Build history of the part. All positions in model axes, mm. Face numbers are marked on the shaded views. A direction names the side the tool comes from. Round coordinates to 2 decimals unless told otherwise and drop trailing zeros. Write each loop counter-clockwise with the first axis right and the second up, starting at its lowest first coordinate (ties: lowest second). Pieces come first, ordered by that corner, then holes. Notation, with made-up numbers: M 10.25,24.5 L 68.25,24.5 A18 ccw 68.25,41.5 Z; hole C -31,-16.75 d5. An arc over 180 degrees is marked long. Write item = value, one per line.
from build123d import *

# Parameters (mm, degrees)
SKETCH1_W           = 80
SKETCH1_H           = 80
BOSS_EXTRUDE1_DEPTH = 60
SKETCH2_W           = 7.262949675
SKETCH2_H           = 50.237294764
CUT_EXTRUDE1_DEPTH  = 83.462112512
SKETCH3_W           = 12.452296607
SKETCH3_H           = 12.893943155
SKETCH3_H_2         = 13.114766428
CUT_EXTRUDE2_DEPTH  = 83.462112512


with BuildPart() as part:
    # Sketch1 → Boss-Extrude1 (new body)
    with BuildSketch(Plane(origin=(0, 0, 0), x_dir=(1, 0, 0), z_dir=(0, 1, 0))):
        Rectangle(SKETCH1_W, SKETCH1_H)
    extrude(amount=BOSS_EXTRUDE1_DEPTH)

    # Sketch2 → Cut-Extrude1 (cut, through all)
    with BuildSketch(Plane(origin=(0, 60, 0), x_dir=(1, 0, 0), z_dir=(0, 1, 0))):
        with Locations((-36.368525163, 0)):
            Rectangle(SKETCH2_W, SKETCH2_H)
    extrude(amount=-CUT_EXTRUDE1_DEPTH, mode=Mode.SUBTRACT)

    # Sketch3 → Cut-Extrude2 (cut, through all)
    with BuildSketch(Plane(origin=(0, 60, 0), x_dir=(1, 0, 0), z_dir=(0, 1, 0))):
        with Locations((33.773851697, 33.553028422)):
            Rectangle(SKETCH3_W, SKETCH3_H)
        with Locations((33.773851697, -33.442616786)):
            Rectangle(SKETCH3_W, SKETCH3_H_2)
    extrude(amount=-CUT_EXTRUDE2_DEPTH, mode=Mode.SUBTRACT)


solid = part.part
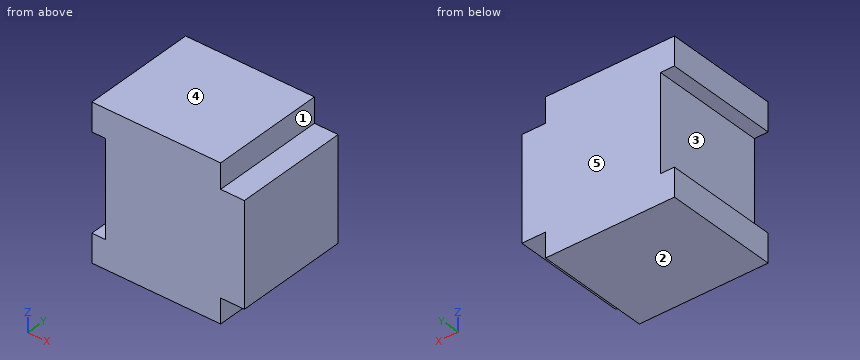
1. Probe probe 1 along X at (y, z) = (28, 31); probe 2 along X at (y, z) = (24, -25). List the from-to ranges inside material, lowest first.
Responses:
probe_1 = -40 to 27.55
probe_2 = -32.74 to 40
2. Tool access for the marked faces 1 and 2: list every direction of +Z, -Z, +X, -X, +Y, -Y with a clear straight run to the whole face (end or side of a thin tool).
Responses:
face_1 = +Z, +X, +Y, -Y
face_2 = -Z, +X, -X, +Y, -Y
3. Band-saw the part on B-B (z = -11). List the corners of the cut face in (x, y).
Responses:
outline = M -32.74,0 L 40,0 L 40,60 L -32.74,60 Z
4. Mould opens along Z. For the marked faces 3, 4 and 5 say: pulls with the +Z half, pulls with the -Z half, needs draft (parallel to the pull), parting line crosses it, or undercut.
Responses:
face_3 = undercut
face_4 = pulls with the +Z half
face_5 = needs draft
5. Band-saw the part on A-A (y = 10). List the corners of the cut face in (x, z).
Responses:
outline = M -40,-40 L 27.55,-40 L 27.55,-27.11 L 40,-27.11 L 40,26.89 L 27.55,26.89 L 27.55,40 L -40,40 L -40,25.12 L -32.74,25.12 L -32.74,-25.12 L -40,-25.12 Z
6. Flat gauge pins, fed straight in: pin 1 (10 mm diameter, centred on y = 7.5, z = 0.5, fed in from -X); pin 2 (6.5 mm diameter, centred on y = 40, z = -36.5, fed in from +X); pin 3 (13.5 mm diameter, centred on x = 35.5, y = 28, fed in from +Z). Where does each tip first touch, or does it go through?
Responses:
pin_1 = -32.74
pin_2 = 27.55
pin_3 = 26.89
